The model under review builds one solid part; all positions refer to its coordinate system, in mm. Face numbers are marked on the shaded views. A direction names the side the tool comes from. Give positions to 0.01 mm unless a question says otherwise; leave off trailing zeros. Loops run counter-clockwise (first coordinate to the right, second up) from the corner with the lowest first, then second, coordinate; pieces in that order, holes last. Notation, with made-up numbers: M 62,-29.5 L 73,-29.5 A5 cw 73,-21.5 Z; hole C 33.5,34 d4. An arc over 180 degrees is marked long. Return JSON: item names as keys, results as strings. Group by question number.
Autodesk Inventor part; units mm, degrees
ref_plane "YZ Plane" through (0, 0, 0) normal (1, 0, 0) x (0, 1, 0)
ref_plane "XZ Plane" through (0, 0, 0) normal (0, 1, 0) x (-1, 0, 0)
ref_plane "XY Plane" through (0, 0, 0) normal (0, 0, 1) x (1, 0, 0)
sketch "スケッチ1" plane through (0, 0, 0) normal (0, 0, 1) x (1, 0, 0)
  circle A0 centre (0, 0) radius 2
  dimension "d0" = 4
extrude "押し出し1" add sketch "スケッチ1" along normal blind 6
sketch "スケッチ2" plane through (0, 0, 6) normal (0, 0, 1) x (1, 0, 0)
  circle A0 centre (0, 0) radius 2
  circle A1 centre (0, 0) radius 4
  dimension "d3" = 8
extrude "押し出し2" add sketch "スケッチ2" along normal blind 3 contours A0 | A1
fillet "フィレット1" radius 3 1 edges at (-4, 0, 9)
thread "ねじ1"
sketch "スケッチ3" plane through (0, 0, 0) normal (0, 0, -1) x (-1, 0, 0)
  circle A0 centre (0, 0) radius 2
extrude "押し出し3" add sketch "スケッチ3" along normal blind 12
properties part number "SB　M4 18mm なべネジ" material "Stainless Steel, 440C"
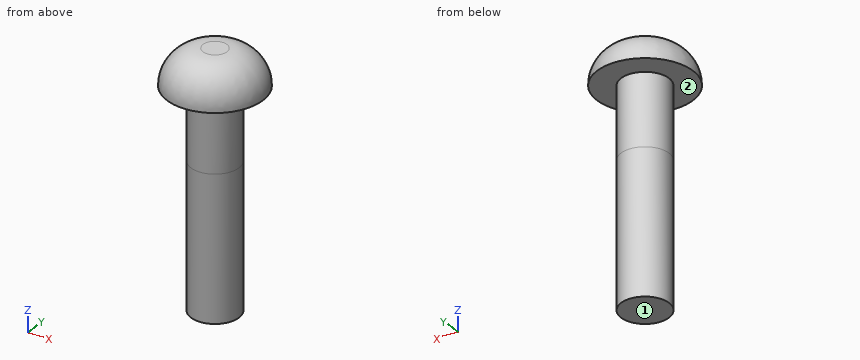
(1) For probe 1 along Z at (x, y) = (-0.5, -1); probe 2 along Z at (x, y) = (2, -0.5); probe 3 along X at (y, z) = (0, 4.25), list the stretches that pass through material, from the lowest coordinate up.
(2) For pin 1 (1.5 mm diameter, centred on x = 1.5, z = 0, fed in from +Y); pin 2 (1.5 mm diameter, centred on x = -2, z = -0.5, fed in from +Y), all flat-tipped, find the tip position at first contact; note any pin that passes through.
(3) For the marked faces 1 and 2, list the 3-axis set-ups (+Z, -Z, +X, -X, +Y, -Y) from which the entire face can be reached by the end or side of a thin tool; tool diameter is ignored.
(4) Add section A-A (z = -8.5). Write out the cut boundary in (x, y), and give its area (3 significant figures).
Verdict:
{
 "1": {"probe 1": "z = -12 to 9", "probe 2": "z = 6 to 8.81", "probe 3": "x = -2 to 2"},
 "2": {"pin 1": "stops at y = 1.85", "pin 2": "stops at y = 1.56"},
 "3": {"face 1": "-Z, +X, -X, +Y, -Y", "face 2": "-Z"},
 "4": {"outline": "C 0,0 d4", "area": "12.6 mm²"}
}
